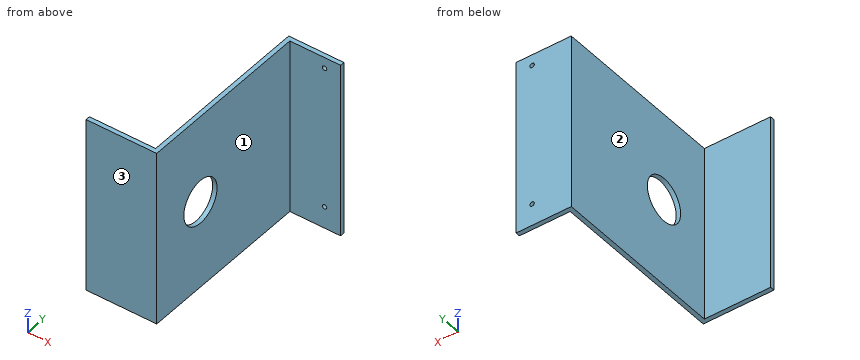
Autodesk Inventor part; units mm, degrees
ref_plane "YZ Plane" through (0, 0, 0) normal (1, 0, 0) x (0, 1, 0)
ref_plane "XZ Plane" through (0, 0, 0) normal (0, 1, 0) x (-1, 0, 0)
ref_plane "XY Plane" through (0, 0, 0) normal (0, 0, 1) x (1, 0, 0)
sketch "Sketch1" plane through (0, 0, 0) normal (0, 1, 0) x (-1, 0, 0)
  line L0 (0, 0) -> (30, 0)
  line L1 (30, 0) -> (30, -80)
  line L2 (30, -80) -> (0, -80)
  line L3 (0, -80) -> (0, 0)
  dimension "d0" = 30
  dimension "d1" = 80
extrude "Extrusion1" add sketch "Sketch1" along normal blind 2
sketch "Sketch2" plane through (0, 0, 0) normal (0, 0, 1) x (1, 0, 0)
  point P0 (0, 0)
sketch "Sketch3" plane through (0, 0, 0) normal (1, 0, 0) x (0, 1, 0)
  line L0 (0, 0) -> (80, 0)
  line L1 (80, 0) -> (80, -80)
  line L2 (80, -80) -> (0, -80)
  line L3 (0, -80) -> (0, 0)
  dimension "d4" = 80
  dimension "d11" = 80
extrude "Extrusion2" add sketch "Sketch3" along normal blind 2
sketch "Sketch4" plane through (0, 0, 0) normal (0, 1, 0) x (-1, 0, 0)
  point P0 (0, 0)
sketch "Sketch5" plane through (0, 0, 0) normal (-1, 0, 0) x (0, 0, 1)
  point P0 (0, 0)
sketch "Sketch6" plane through (0, 80, 0) normal (0, 1, 0) x (1, 0, 0)
  line L0 (-30, 0) -> (0, 0)
  line L1 (0, 0) -> (25, 0)
  line L2 (25, 0) -> (25, 80)
  line L3 (25, 80) -> (0, 80)
  line L4 (0, 80) -> (0, 0)
  dimension "d7" = 25
  dimension "d8" = 80
extrude "Extrusion3" add sketch "Sketch6" along normal blind 2
sketch "Sketch7" plane through (0, 2, 0) normal (0, 1, 0) x (1, 0, 0)
  point P0 (0, 0)
  point P1 (-20.3201, 56.529)
  point P2 (-18.421, 5.5073)
sketch "Sketch8" plane through (0, 0, 0) normal (0, -1, 0) x (1, 0, 0)
  point P0 (0, 0)
sketch "Sketch9" plane through (0, 80, 0) normal (0, -1, 0) x (1, 0, 0)
  line L0 (2, -80) -> (2, 0)
  line L1 (2, 0) -> (25, 0)
  line L2 (25, -80) -> (2, -80)
  point P0 (0, 0)
  point P1 (2, -65)
  point P2 (2, 0)
  point P3 (17.7309, -70)
  point P4 (2, 0)
  point P5 (17.7309, 0)
  point P6 (17.7309, -70)
  point P7 (17.7309, -5)
  dimension "d12" = 10
hole "Hole1" at (17.7309, 80, -70) at (17.7309, 80, -5) direction (0, 1, 0) diameter 2 depth 25 tip angle 118
sketch "Sketch10" plane through (2, 0, 0) normal (1, 0, 0) x (0, 0, -1)
  circle A0 centre (40, 26.2693) radius 10
  line L0 (80, 0) -> (80, 80)
  point P0 (0, 0)
  dimension "d20" = 20
  dimension "d21" = 40
extrude "Extrusion4" cut sketch "Sketch10" against normal blind 2
sketch "Sketch11" plane through (2, 0, 0) normal (1, 0, 0) x (0, 0, -1)
  point P0 (0, 0)
sketch "Sketch12" plane through (0, 0, 0) normal (-1, 0, 0) x (0, 0, 1)
  point P0 (0, 0)
properties part number "dc clamp" material "Lead"
Here's how the part is built. I have some questions about the finished solid (model axes, mm). Face numbers are marked on the shaded views. A direction names the side the tool comes from. Give positions to 0.01 mm unless a question says otherwise; leave off trailing zeros. Loops run counter-clockwise (first coordinate to the right, second up) from the corner with the lowest first, then second, coordinate; pieces in that order, holes last. Notation, with made-up numbers: M -31,-20.5 L -14,-20.5 A16 cw -14,-1.5 Z; hole C -23.5,67.5 d4. An arc over 180 degrees is marked long. Return JSON: item names as keys, results as strings.
Item 1: Imagine slicing it at B-B on y = 20. List the corners of the cut face in (x, z) for me.
A:
{"outline": "M 0,-80 L 2,-80 L 2,-47.79 L 0,-47.79 Z; M 0,-32.21 L 2,-32.21 L 2,0 L 0,0 Z"}
Item 2: Imagine slicing it at C-C on z = -18.5. List the corners of the cut face in (x, y) for me, then the cut area to 3 significant figures.
A:
{"outline": "M -30,0 L 2,0 L 2,80 L 25,80 L 25,82 L 0,82 L 0,2 L -30,2 Z", "area": "270 mm^2"}
Item 3: Imagine slicing it at D-D on x = -25. List the corners of the cut face in (y, z) for me, then the cut area to 3 significant figures.
A:
{"outline": "M 0,-80 L 2,-80 L 2,0 L 0,0 Z", "area": "160 mm^2"}
Item 4: On a 3-axis mill with a long thin cutter (end or side, diameter ignored), from which of +Z, -Z, +X, -X, +Y, -Y can I reach the whole of each face in a straight line? I mean the marked faces 1, 2 and 3. Say none if no direction works.
A:
{"face 1": "+Z, -Z, +X, -Y", "face 2": "+Z, -Z, -X, +Y", "face 3": "+Z, -Z, +X, -X, -Y"}
Item 5: I'm going to push flat-ended pins straight in: pin 1 Ø2.5 at (x, z) = (17.73, -70) entering from -Y; pin 2 Ø4 at (x, z) = (-13, -37.5) entering from -Y; pin 3 Ø10 at (y, z) = (17, -21) entering from +X; pin 4 Ø15 at (x, z) = (-14, -50.5) entering from +Y. Where does each tip first touch, or does it pass through?
A:
{"pin 1": "stops at y = 80", "pin 2": "stops at y = 0", "pin 3": "stops at x = 2", "pin 4": "stops at y = 2"}
Item 6: Imagine slicing it at A-A on z = -40. List the corners of the cut face in (x, y) for me, then the cut area to 3 significant figures.
A:
{"outline": "M -30,0 L 2,0 L 2,16.27 L 0,16.27 L 0,2 L -30,2 Z; M 0,36.27 L 2,36.27 L 2,80 L 25,80 L 25,82 L 0,82 Z", "area": "230 mm^2"}
Item 7: Please list where these lines run through material, in increasing order: line 1 (Y direction, x = 8.5, z = -61); line 2 (X direction, y = 57, z = -68).
A:
{"line 1": "y = 80 to 82", "line 2": "x = 0 to 2"}
